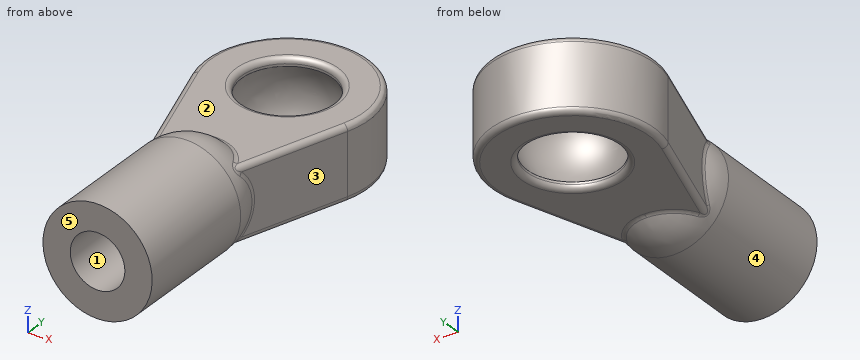
```python
from build123d import *

# Parameters (mm, degrees)
BOSS_EXTRU_1_DEPTH      = 2
BOSS_EXTRU_1_DEPTH_BACK = 2
ESQUISSE2_R             = 2.5
CONG_1_R                = 0.3


with BuildPart() as part:
    # Esquisse1 → R_volution1 (revolve)
    with BuildSketch(Plane.XY, mode=Mode.PRIVATE) as r_volution1_sk:
        with BuildLine():
            Line((0, 6), (0, 10))
            ThreePointArc((0, 10), (-2.121320344, 9.121320344), (-3, 7))
            Line((-3, 7), (-3, 0))
            Line((-3, 0), (-1.5, 0))
            Line((-1.5, 0), (-1.5, 6))
            Line((-1.5, 6), (0, 6))
        make_face()
    revolve(r_volution1_sk.sketch.rotate(Axis((0, -0.674983233, 0), (0, 1, 0)), 270), axis=Axis((0, -0.674983233, 0), (0, 1, 0)))

    # Esquisse2 → Boss.-Extru.1 (add, two sides: drawn at the far end of the back side and taken through both)
    with BuildSketch(Plane.XY.offset(-BOSS_EXTRU_1_DEPTH_BACK)):
        with BuildLine():
            Line((-2.132222439, 7), (-4.279754323, 13.609423525))
            ThreePointArc((-4.279754323, 13.609423525), (0, 19.5), (4.279754323, 13.609423525))
            Line((4.279754323, 13.609423525), (2.132222439, 7))
            Line((2.132222439, 7), (-2.132222439, 7))
        make_face()
        with Locations((0, 15)):
            Circle(ESQUISSE2_R, mode=Mode.SUBTRACT)
    extrude(amount=BOSS_EXTRU_1_DEPTH + BOSS_EXTRU_1_DEPTH_BACK)

    # Esquisse3 → Enl_vement de mati_re-R_volution1 (revolve, cut)
    with BuildSketch(Plane.XY):
        with BuildLine():
            Line((0, 17.95), (0, 12.05))
            ThreePointArc((0, 12.05), (-2.95, 15), (0, 17.95))
        make_face()
    revolve(axis=Axis((0, 11.065209796, 0), (0, 1, 0)), mode=Mode.SUBTRACT)

    # Cong_1
    cong_1_edges = [part.edges().sort_by_distance(p)[0] for p in [
        (-3.249763904, 10.439438968, -2),
        (0, 19.5, -2),
        (3.249763904, 10.439438968, -2),
        (-2.5, 15, -2),
        (-2.5, 15, 2),
        (3.249763904, 10.439438968, 2),
        (0, 19.5, 2),
        (-3.249763904, 10.439438968, 2),
    ]]
    fillet(cong_1_edges, radius=CONG_1_R)
    cong_1_2_edges = [part.edges().sort_by_distance(p)[0] for p in [
        (2.4e-08, 9.236067977, 2),
        (2.611797225, 8.475979423, 3.5e-08),
        (-2.611797225, 8.475979423, -3.5e-08),
        (-1.260069045, 8.847221157, -2),
        (1.260069046, 8.847221156, -2),
        (2.233299855, 7.596099057, -1.912338273),
        (-2.233299855, 7.596099057, -1.912338273),
        (-2.233315922, 7.596093395, 1.912321273),
        (2.233315922, 7.596093395, 1.912321273),
    ]]
    fillet(cong_1_2_edges, radius=CONG_1_R)


solid = part.part
```
Check sheet for the modelled part. Datum: model origin and axes. Units: mm. Face numbers are marked on the shaded views. A direction names the side the tool comes from. Give positions to 0.01 mm unless a question says otherwise; leave off trailing zeros. Return JSON: item names as keys, results as strings.
1. Go/stop test with flat-tipped pins: P1, Ø4.5, axis at x = 0, y = 15, coming from the +Z side; P2, Ø1.5, axis at x = 2, z = 0, coming from the -Y side; P3, Ø1, axis at y = 7.5, z = 1, coming from the +X side. Record where each tip stops, or that it passes through.
From the geometry:
{"P1": "through", "P2": "y = 0", "P3": "x = 2.94"}
2. Material ranges on probe 1 along X at (y, z) = (15, 1.65); probe 2 along Y at (x, z) = (1.25, 0.7); probe 3 along Y at (x, z) = (-2, -1.65), recorded low to high. Write a range as [from, to].
From the geometry:
{"probe 1": "[-4.5, -2.5], [2.5, 4.5]", "probe 2": "[6, 12.42], [17.58, 19.32]", "probe 3": "[0, 13.5], [16.5, 19.03]"}
3. Set-up check for the marked faces 4 and 5: record each of +Z, -Z, +X, -X, +Y, -Y from which the full face is reachable in a straight line by a thin tool's end or side.
From the geometry:
{"face 4": "-Y", "face 5": "+Z, -Z, +X, -X, -Y"}
4. Mould release check, pull along Z, two halves, no side actions. Record for the marked faces 1, 2 and 3: +Z half, -Z half, draft (parallel to the pull), parting line (faces both ways), or undercut.
From the geometry:
{"face 1": "undercut", "face 2": "+Z half", "face 3": "draft"}
